Autodesk Inventor part; units mm, degrees
ref_plane "YZ Plane" through (0, 0, 0) normal (1, 0, 0) x (0, 1, 0)
ref_plane "XZ Plane" through (0, 0, 0) normal (0, 1, 0) x (-1, 0, 0)
ref_plane "XY Plane" through (0, 0, 0) normal (0, 0, 1) x (1, 0, 0)
sketch "Sketch1" plane through (0, 0, 0) normal (0, 1, 0) x (-1, 0, 0)
  circle A0 centre (0, 0) radius 152.4
  circle A1 centre (0, 0) radius 165.1
  dimension "d0" = 304.8
  dimension "d1" = 330.2
extrude "Extrusion1" add sketch "Sketch1" along normal blind 152.4
sketch "Sketch2" plane through (0, 0, 0) normal (1, 0, 0) x (0, 1, 0)
  circle A0 centre (100.6077, 0) radius 25.4
  point P0 (0, 0)
  dimension "d4" = 50.8
extrude "Extrusion2" add sketch "Sketch2" along normal mid plane 889
sketch "Sketch4" plane through (0, 152.4, 0) normal (0, 1, 0) x (1, 0, 0)
  circle A0 centre (0, 0) radius 152.4
extrude "Extrusion4" cut sketch "Sketch4" against normal through all
sketch "Sketch5" plane through (0, 152.4, 0) normal (0, 1, 0) x (1, 0, 0)
  circle A0 centre (0, 0) radius 165.1
extrude "Extrusion5" add sketch "Sketch5" along normal blind 50.8 draft -50
sketch "Sketch6" plane through (0, 152.4, 0) normal (0, -1, 0) x (1, 0, 0)
  circle A0 centre (0, 0) radius 104.5589
  circle A1 centre (0, 0) radius 50.8
  dimension "d15" = 101.6
extrude "Extrusion6" add sketch "Sketch6" along normal blind 863.6 contours A1
sketch "Sketch7" plane through (0, -711.2, 0) normal (0, -1, 0) x (1, 0, 0)
  circle A0 centre (0, 0) radius 104.5589
  circle A1 centre (0, 0) radius 101.6
  dimension "d18" = 203.2
extrude "Extrusion7" add sketch "Sketch7" along normal blind 25.4 contours A1
ref_plane "Work Plane1" through (0, -609.6, 0) normal (0, 1, 0) x (1, 0, 0)
sketch "Sketch8" plane through (0, -609.6, 0) normal (0, 1, 0) x (1, 0, 0)
  circle A0 centre (0, 0) radius 101.6
  dimension "d22" = 203.2
extrude "Extrusion8" add sketch "Sketch8" along normal blind 25.4
ref_plane "Work Plane2" through (75.376, -18.8821, -44.9646) normal (1, 0, 0) x (0, 1, 0)
sketch "Sketch9" plane through (75.376, -18.8821, -44.9646) normal (1, 0, 0) x (0, 1, 0)
  circle A0 centre (-604.603, 44.9646) radius 12.7
  point P0 (18.8821, 44.9646)
  dimension "d25" = 25.4
extrude "Extrusion9" cut sketch "Sketch9" against normal through all
properties part number "capistan upper"
Check sheet for the modelled part. Datum: model origin and axes. Units: mm. A direction names the side the tool comes from. Round coordinates to 2 decimals unless told otherwise and drop trailing zeros. Write each loop counter-clockwise with the first axis right and the second up, starting at its lowest first coordinate (ties: lowest second). Pieces come first, ordered by that corner, then holes. Notation, with made-up numbers: (20, 24) -> (69, 24) arc R27 ccw to (69, 47) -> close; hole circle Ø9 at (88.25, 72.25). An arc over 180 degrees is marked (long way). One line per question, with ' | ' between items. Start each with the question number.
1. Set-up check for faces 1 (the face through (-1, -736.6, 1)), 2 (the face through (-144.985, 75.133, -46.957)), 3 (the face through (48.454, -659.689, -15.259)), 4 (the face through (301.847, 124.835, -7.629)): record each of +Z, -Z, +X, -X, +Y, -Y from which the full face is reachable in a straight line by a thin tool's end or side.
2. Sectioned sample at B-B, the plane y = 25. Record the cut outline in (x, z), then the cut area to 3 significant figures.
3. Sectioned sample at A-A, the plane x = 0. Record the cut outline in (y, z), then the cut area to 3 significant figures.
4. Sectioned sample at C-C, the plane z = -82.5. Count the separate pieces of the cut face and the enclosed holes in it, then the cut area to 3 significant figures.
5. Release check for a two-part mould opening along Y. For faces 5 (the face through (-22.025, -597.078, -99.184)), 6 (the face through (66, 152.4, -2)), 7 (the face through (-1, 203.2, -1)), 8 (the face through (-301.847, 124.835, 7.629)) record: +Y half, -Y half, draft (parallel to the pull), parting line (faces both ways), or undercut.
6. Depth check by flat-ended pin: pin 1 (8 mm diameter, centred on x = -201, z = 18, fed in from -Y); pin 2 (8 mm diameter, centred on x = -110, y = 67, fed in from -Z); pin 3 (4 mm diameter, centred on x = 320, z = -7.5, fed in from +Y). Enter the tip coordinate at first touch or a pass-through.
7. Sectioned sample at D-D, the plane x = 279.5. Record the cut outline in (y, z).
8. Scan lines: line 1 along Z through (x, y) = (0, 31.5); line 2 along X through (y, z) = (90, 0). Record each from-to range of solid material in increasing order. Write a range as from..to.
Taken from the geometry:
1) face 1: +Z, -Z, +X, -X, -Y | face 2: -Y | face 3: none | face 4: +X
2) outline: circle Ø330.2 at (0, 0); circle Ø101.6 at (0, 0); hole circle Ø304.8 at (0, 0) | area: 20,800 mm^2
3) outline: (-736.6, -101.6) -> (-711.2, -101.6) -> (-711.2, -50.8) -> (-609.6, -50.8) -> (-609.6, -101.6) -> (-584.2, -101.6) -> (-584.2, -50.8) -> (152.4, -50.8) -> (152.4, -152.4) -> (0, -152.4) -> (0, -165.1) -> (152.4, -165.1) -> (203.2, -104.56) -> (203.2, 104.56) -> (152.4, 165.1) -> (0, 165.1) -> (0, 152.4) -> (152.4, 152.4) -> (152.4, 50.8) -> (-584.2, 50.8) -> (-584.2, 101.6) -> (-609.6, 101.6) -> (-609.6, 50.8) -> (-711.2, 50.8) -> (-711.2, 101.6) -> (-736.6, 101.6) -> close; hole circle Ø25.4 at (-623.49, 0) | area: 113,000 mm^2
4) separate pieces: 3 | enclosed holes: 0 | area: 21,300 mm^2
5) face 5: draft | face 6: undercut | face 7: +Y half | face 8: parting line
6) pin 1: stops at y = 79.41 | pin 2: stops at z = -126.58 | pin 3: stops at y = 125.41
7) outline: circle Ø50.8 at (100.61, 0)
8) line 1: z = -165.1..-152.4, -50.8..50.8, 152.4..165.1 | line 2: x = -444.5..-152.4, -50.8..50.8, 152.4..444.5
